Study the drawing (mm; zero at the part's minimum x, y, z) and answer. A direction names the side the tool comes from. Give positions to 0.01 mm unless a question says otherwise; leave off trailing zeros. Write each loop counter-clockwise with the first axis right and the second up, starting at its lowest first coordinate (ties: lowest second). Pieces come first, ordered by that corner, then holes. Notation, with made-up numbers: (79, 24) - (132, 24) arc R18 ccw to (132, 56) - close; hole circle Ø3 at (87, -4). An arc over 180 degrees is marked (long way). Return JSON: item names as keys, results as strings.
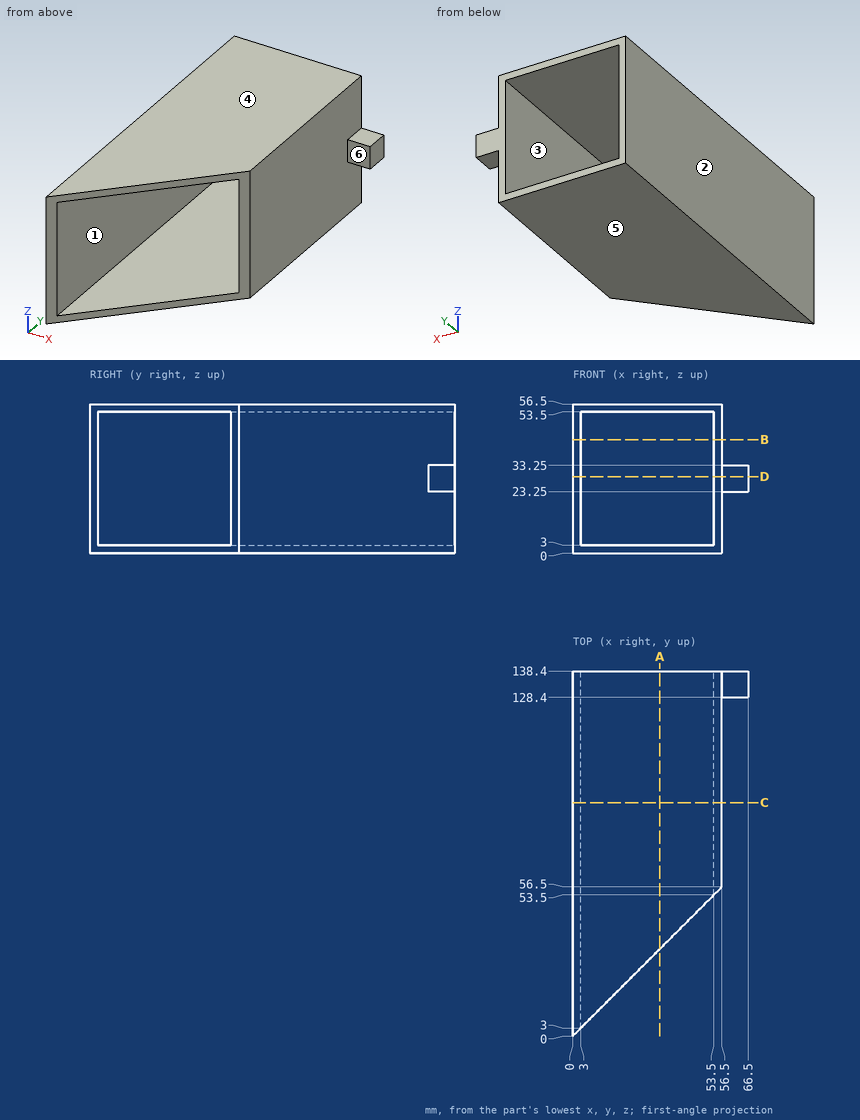
Item 1: The mould has two halves that part along Z. Classify the marked faces 3, 4, 5 and 6: +Z half, -Z half, draft (parallel to the pull), parting line (faces both ways), or undercut.
Answer below:
{"face 3": "undercut", "face 4": "+Z half", "face 5": "-Z half", "face 6": "draft"}
Item 2: Consider L1, parallel to X at y = 126.5, z = 49; L2, parallel to X at y = 39, z = 19. Determine where each line is inside the solid, lowest interval first.
Answer below:
{"L1": "x = 0 to 3, 53.5 to 56.5", "L2": "x = 0 to 3"}
Item 3: A cutting plane is placed at C-C on y = 88.5. Determine the outline of the cut face in (x, z).
Answer below:
{"outline": "(0, 0) - (56.5, 0) - (56.5, 56.5) - (0, 56.5) - close; hole (3, 3) - (53.5, 3) - (53.5, 53.5) - (3, 53.5) - close"}
Item 4: A cutting plane is placed at D-D on z = 29. Determine the outline of the cut face in (x, y).
Answer below:
{"outline": "(0, 0) - (3, 3) - (3, 138.4) - (0, 138.4) - close; (53.5, 53.5) - (56.5, 56.5) - (56.5, 128.4) - (66.5, 128.4) - (66.5, 138.4) - (53.5, 138.4) - close"}
Item 5: A cutting plane is placed at B-B on z = 43. Determine the outline of the cut face in (x, y), then the cut area to 3 significant figures.
Answer below:
{"outline": "(0, 0) - (3, 3) - (3, 138.4) - (0, 138.4) - close; (53.5, 53.5) - (56.5, 56.5) - (56.5, 138.4) - (53.5, 138.4) - close", "area": "661 mm²"}
Item 6: A cutting plane is placed at A-A on x = 33. Determine the outline of the cut face in (y, z), then the cut area to 3 significant figures.
Answer below:
{"outline": "(33, 0) - (138.4, 0) - (138.4, 3) - (33, 3) - close; (33, 53.5) - (138.4, 53.5) - (138.4, 56.5) - (33, 56.5) - close", "area": "632 mm²"}
Item 7: For the marked faces 1 and 2, determine the directions among +Z, -Z, +X, -X, +Y, -Y from which every point of the face is accessible in a straight line to the end or side of a thin tool.
Answer below:
{"face 1": "+Y, -Y", "face 2": "+Z, -Z, -X, +Y, -Y"}
Item 8: A flat-ended cylindrical pin translates along its axis: P1, Ø17, axis at y = 82.5, z = 15, coming from the +X side. Find the tip coordinate at first contact, or state that the pin passes through.
Answer below:
{"P1": "stops at x = 56.5"}
